Autodesk Inventor part; units mm, degrees
ref_plane "YZ Plane" through (0, 0, 0) normal (1, 0, 0) x (0, 1, 0)
ref_plane "XZ Plane" through (0, 0, 0) normal (0, 1, 0) x (-1, 0, 0)
ref_plane "XY Plane" through (0, 0, 0) normal (0, 0, 1) x (1, 0, 0)
sketch "Szkic1" plane through (0, 0, 0) normal (0, 0, 1) x (1, 0, 0)
  line L0 (-40, -25.5) -> (40, -25.5)
  line L1 (40, -25.5) -> (40, 25.5)
  line L2 (40, 25.5) -> (-40, 25.5)
  line L3 (-40, 25.5) -> (-40, -25.5)
  line L4 (22.5, 0) -> (22.5, 25.5)
  line L5 (22.5, 25.5) -> (-22.5, 25.5)
  line L6 (-22.5, -25.5) -> (22.5, -25.5)
  line L7 (-29.5, -15) -> (-29.5, 15) construction
  line L8 (-27.5, -15) -> (-27.5, 15)
  line L9 (-31.5, 15) -> (-31.5, -15)
  arc A0 (-31.5, -15) -> (-27.5, -15) centre (-29.5, -15) ccw
  arc A1 (-27.5, 15) -> (-31.5, 15) centre (-29.5, 15) ccw
  line L10 (29.5, -15) -> (29.5, 15) construction
  line L11 (31.5, -15) -> (31.5, 15)
  line L12 (27.5, 15) -> (27.5, -15)
  arc A2 (27.5, -15) -> (31.5, -15) centre (29.5, -15) ccw
  arc A3 (31.5, 15) -> (27.5, 15) centre (29.5, 15) ccw
  line L13 (27.5, 0) -> (29.5, 0)
  arc A4 (-22.5, 0) -> (22.5, 0) centre (0, 0) ccw
  line L14 (-22.5, 25.5) -> (-22.5, 0)
  line L15 (37, -22) -> (-37, -22)
  line L16 (-37, -22) -> (-37, 22)
  line L17 (-37, 22) -> (37, -22) construction
  line L18 (37, 22) -> (-37, -22) construction
  circle A5 centre (-37, -22) radius 1
  circle A6 centre (-37, -22) radius 2
  circle A7 centre (37, -22) radius 2
  circle A8 centre (37, -22) radius 1
  circle A9 centre (-37, 22) radius 2
  circle A10 centre (-37, 22) radius 1
  circle A11 centre (37, 22) radius 2
  circle A12 centre (37, 22) radius 1
  dimension "d1" = 51
  dimension "d14" = 4
  dimension "d15" = 15
  dimension "d16" = 4
  dimension "d26" = 44
  dimension "d27" = 2
  dimension "d28" = 4
  dimension "d31" = 74
  dimension "d34" = 44
extrude "Wyciągnięcie proste1" add sketch "Szkic1" along normal blind 1.5 contours L3 L2 L14 A4 L4 L1 L0 | A6 L16 A5 L15 | L15 A5 L16 A6 | A7 | A9 | A11
extrude "Wyciągnięcie proste2" add sketch "Szkic1" against normal blind 8 contours A6 L16 A5 L15 | L15 A5 L16 A6 | A7 | A9 | A11
fillet "Zaokrąglenie1" radius 2 3 edges at (-22.5, 12.75, 0) (22.5, 12.75, 0) (0, -22.5, 0)
properties part number "FrontHolder"
Here's how the part is built. I have some questions about the finished solid (model axes, mm). A direction names the side the tool comes from. Give positions to 0.01 mm unless a question says otherwise; leave off trailing zeros. Loops run counter-clockwise (first coordinate to the right, second up) from the corner with the lowest first, then second, coordinate; pieces in that order, holes last. Notation, with made-up numbers: (-8, 58.25) -> (7, 58.25) arc R18 ccw to (7, 69.25) -> close; hole circle Ø5 at (60, 74.5). An arc over 180 degrees is marked (long way). One line per item, written item: value.
Q1. Suppose I cut it at C-C on x = 29.5. Please give me the cut outline in (y, z).
Answers follow:
outline: (-25.5, 0) -> (-17, 0) -> (-17, 1.5) -> (-25.5, 1.5) -> close; (17, 0) -> (25.5, 0) -> (25.5, 1.5) -> (17, 1.5) -> close
Q2. If I drill on line 1 along Y through (x, z) = (-37, -0.25); line 2 along X through (y, z) = (-22, -2.75); line 3 along X through (y, z) = (11.5, 1), over which ranges is the centre line in solid material (lowest first)?
Answers follow:
line 1: -24 to -23, -21 to -20, 20 to 21, 23 to 24
line 2: -39 to -38, -36 to -35, 35 to 36, 38 to 39
line 3: -40 to -31.5, -27.5 to -22.7, 22.7 to 27.5, 31.5 to 40
Q3. We'd pull the mould along Y, two halves only. Please class faces 1 (the face through (-1, -25.5, 1)), 2 (the face through (23.2, 12.57, 0.43)), 3 (the face through (-38.474, -20.648, -3.944)): pulls with the +Y half, pulls with the -Y half, needs draft (parallel to the pull), parting line crosses it, or undercut.
Answers follow:
face 1: pulls with the -Y half
face 2: needs draft
face 3: undercut
Q4. I'm going to push flat-ended pins straight in: pin 1 Ø3 at (x, z) = (20, -2) entering from +Y; pin 2 Ø1 at (y, z) = (20, -1) entering from -X. Where does each tip first touch, or does it pass through?
Answers follow:
pin 1: through
pin 2: x = -38.32
Q5. Suppose I cut it at B-B on y = 18. Please give me the cut outline in (x, z).
Answers follow:
outline: (-40, 0) -> (-24.44, 0) arc R2 ccw to (-22.5, 1.5) -> (-40, 1.5) -> close; (22.5, 1.5) arc R2 ccw to (24.44, 0) -> (40, 0) -> (40, 1.5) -> close
Q6. On a 3-axis mill with a long thin cutter (end or side, diameter ignored), from which of +Z, -Z, +X, -X, +Y, -Y can I reach the whole of each face in a straight line? I mean faces 4 (the face through (-23.2, 12.93, 0.43)), 5 (the face through (29.5, -17, 0.7)), 6 (the face through (38.847, 21.234, -3.944)). Say none if no direction works.
Answers follow:
face 4: -Z, +Y
face 5: +Z, -Z
face 6: -Z
Q7. Suppose I cut it at A-A on z = -4.5. Please give me the cut outline in (x, y), then the cut area to 3 significant figures.
Answers follow:
outline: circle Ø4 at (-37, -22); circle Ø4 at (-37, 22); circle Ø4 at (37, -22); circle Ø4 at (37, 22); hole circle Ø2 at (-37, -22); hole circle Ø2 at (-37, 22); hole circle Ø2 at (37, -22); hole circle Ø2 at (37, 22)
area: 37.7 mm^2
